```python
from build123d import *

# Parameters (mm, degrees)
BOSS_EXTRUDE1_DEPTH = 6.35
FILLET1_R           = 5.08


with BuildPart() as part:
    # Sketch2 → Boss-Extrude1 (new body)
    with BuildSketch(Plane.XY):
        with BuildLine():
            Line((-5.12438972, 14.653837172), (267.16361028, 14.653837172))
            ThreePointArc((267.16361028, 14.653837172), (268.959661504, 15.397785947), (269.70361028, 17.193837172))
            Line((269.70361028, 17.193837172), (269.70361028, 75.613837172))
            ThreePointArc((269.70361028, 75.613837172), (268.959661504, 77.409888396), (267.16361028, 78.153837172))
            Line((267.16361028, 78.153837172), (-5.12438972, 78.153837172))
            ThreePointArc((-5.12438972, 78.153837172), (-6.920440944, 77.409888396), (-7.66438972, 75.613837172))
            Line((-7.66438972, 75.613837172), (-7.66438972, 17.193837172))
            ThreePointArc((-7.66438972, 17.193837172), (-6.920440944, 15.397785947), (-5.12438972, 14.653837172))
        make_face()
        Polygon((30.05461028, 24.406794359), (4.65461028, 68.400884872), (55.45461028, 68.400884872), align=None, mode=Mode.SUBTRACT)
        Polygon((70.44061028, 68.400882428), (95.84061028, 24.406791915), (45.04061028, 24.406791915), align=None, mode=Mode.SUBTRACT)
        Polygon((110.82627023, 24.305837172), (85.42627023, 68.299927684), (136.22627023, 68.299927684), align=None, mode=Mode.SUBTRACT)
        Polygon((125.81227023, 24.305834728), (151.21227023, 68.29992524), (176.61227023, 24.305834728), align=None, mode=Mode.SUBTRACT)
        Polygon((191.59793018, 24.204879984), (166.19793018, 68.198970496), (216.99793018, 68.198970496), align=None, mode=Mode.SUBTRACT)
        Polygon((206.58393018, 24.20487754), (231.98393018, 68.198968052), (257.38393018, 24.20487754), align=None, mode=Mode.SUBTRACT)
    extrude(amount=BOSS_EXTRUDE1_DEPTH)

    # Fillet1
    fillet1_edges = [part.edges().sort_by_distance(p)[0] for p in [
        (257.38393018, 24.20487754, 3.175),
        (231.98393018, 68.198968052, 3.175),
        (206.58393018, 24.20487754, 3.175),
        (176.61227023, 24.305834728, 3.175),
        (151.21227023, 68.29992524, 3.175),
        (125.81227023, 24.305834728, 3.175),
        (4.65461028, 68.400884872, 3.175),
        (30.05461028, 24.406794359, 3.175),
        (55.45461028, 68.400884872, 3.175),
        (95.84061028, 24.406791915, 3.175),
        (70.44061028, 68.400882428, 3.175),
        (45.04061028, 24.406791915, 3.175),
        (85.42627023, 68.299927684, 3.175),
        (110.82627023, 24.305837172, 3.175),
        (136.22627023, 68.299927684, 3.175),
        (166.19793018, 68.198970496, 3.175),
        (191.59793018, 24.204879984, 3.175),
        (216.99793018, 68.198970496, 3.175),
    ]]
    fillet(fillet1_edges, radius=FILLET1_R)


solid = part.part
```
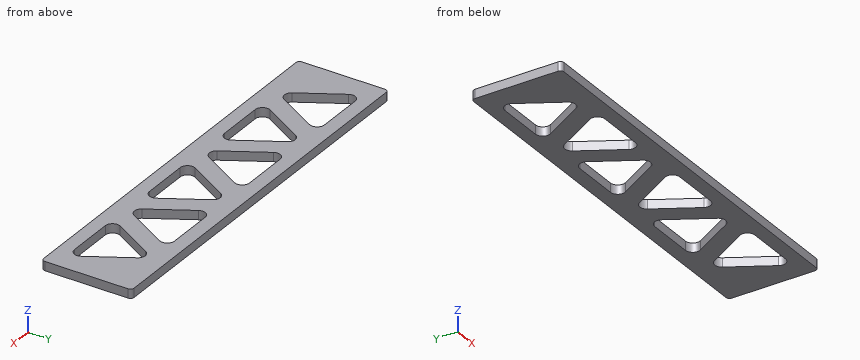
For this review, take the finished solid that the model builds, in its own axes (mm). Coordinates: 2 decimals unless noted, no trailing zeros. Order: outer loops, then holes, each group sorted by start corner. A loop starts at its lowest first (then second) coordinate and runs counter-clockwise, first axis right, second up. Notation, with made-up numbers: (39.25, 30.5) -> (84.25, 30.5) arc R30 ccw to (84.25, 61.5) -> close; hole circle Ø1 at (8.25, 31.25). An arc over 180 degrees is marked (long way). Answer as CSV lines item,"result".
Q1. Wall thickness on line 1 along Y through (x, z) = (110, 2); line 2 along X through (y, z) = (64.5, 5.25); line 3 along X through (y, z) = (66, 5.25): over which ranges is each line inside the solid? List them lowest first. Write a range as [from, to].
Model answer:
line 1,"y = [14.65, 29.45], [68.3, 78.15]"
line 2,"x = [-7.66, 8.51], [51.6, 89.31], [132.34, 170.11], [213.09, 269.7]"
line 3,"x = [-7.66, 9.14], [50.97, 89.97], [131.68, 170.81], [212.38, 269.7]"
Q2. We need section A-A (y = 36). State the section outline as (x, z) points, plus the area to 3 significant figures.
Model answer:
outline,"(-7.66, 0) -> (23.36, 0) -> (23.36, 6.35) -> (-7.66, 6.35) -> close; (36.75, 0) -> (51.73, 0) -> (51.73, 6.35) -> (36.75, 6.35) -> close; (89.15, 0) -> (104.07, 0) -> (104.07, 6.35) -> (89.15, 6.35) -> close; (117.58, 0) -> (132.56, 0) -> (132.56, 6.35) -> (117.58, 6.35) -> close; (169.86, 0) -> (184.79, 0) -> (184.79, 6.35) -> (169.86, 6.35) -> close; (198.41, 0) -> (213.39, 0) -> (213.39, 6.35) -> (198.41, 6.35) -> close; (250.57, 0) -> (269.7, 0) -> (269.7, 6.35) -> (250.57, 6.35) -> close"
area,"794 mm2"
Q3. Clearance check with a flat-ended pin moving along its axis: pin 1 Ø5 at (x, y) = (181, 71) entering from -Z. State where the tip first meets the part, or that it passes through.
Model answer:
pin 1,"stops at z = 0"
Q4. We need section B-B (x = 242). State the section outline as (y, z) points, plus the area to 3 significant figures.
Model answer:
outline,"(14.65, 0) -> (24.2, 0) -> (24.2, 6.35) -> (14.65, 6.35) -> close; (50.85, 0) -> (78.15, 0) -> (78.15, 6.35) -> (50.85, 6.35) -> close"
area,"234 mm2"
Q5. We need section C-C (z = 4.75). Count the separate pieces of the cut face and the enclosed holes in it, plus the area to 3 significant figures.
Model answer:
separate pieces,"1"
enclosed holes,"6"
area,"11,200 mm2"
